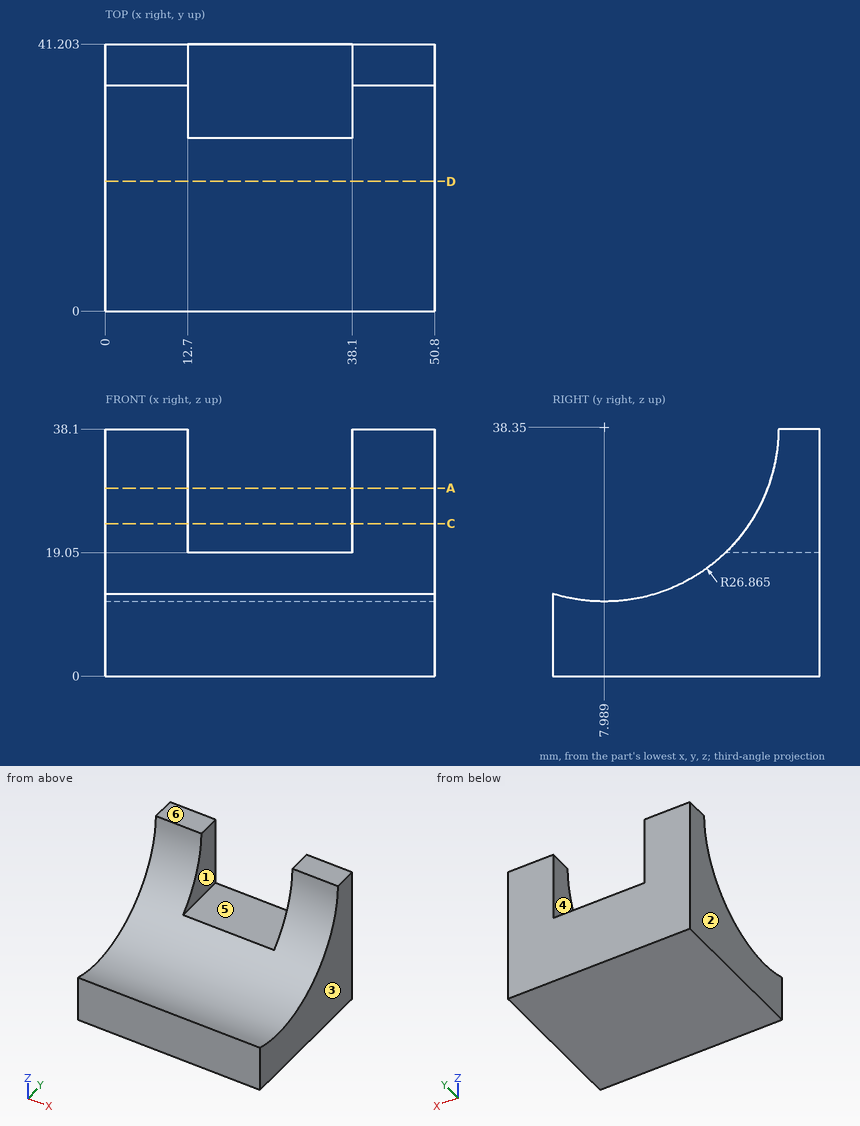
Geometry: see drawing. Coordinates: mm, zero at the bounding-box minimum. A direction names the side the tool comes from. Give positions to 0.01 mm unless a question says otherwise; leave off trailing zeros. Loops run counter-clockwise (first coordinate to the right, second up) from the corner with the lowest first, then second, coordinate; pieces in that order, holes last. Notation, with made-up numbers: M 79.5,88 L 128.5,88 A21 ccw 128.5,110 Z; hole C 67.5,24.25 d11. An arc over 180 degrees is marked long. Answer as CSV lines item,"result". Start each with the question number.
1. Pin query (flat end, axial travel): P1, Ø11.5, axis at x = 29, y = 33, coming from the +Z side. Return the tip coordinate at first contact, or that it passes through.
2. Pull-direction query (X, two-part tool) for the marked faces 3, 4, 5 and 6; classes: released by +X, released by -X, zero draft, split by the parting line, or undercut.
3. Reachability of the marked faces 1 and 2 from +Z, -Z, +X, -X, +Y, -Y: full face, straight path, thin tool, end or side. Return the list, or none.
4. Section A-A on z = 29. Return loops of the section in (x, y) (1 decimal), plus the area to 3 significant figures.
5. Line query: L1, parallel to X at y = 33, z = 26; L2, parallel to Z at x = 36, y = 33.5; L3, parallel to Z at x = 38.5, y = 7.5. Output: solid intervals per line, ascending.
6. Section C-C on z = 23.5. Return loops of the section in (x, y), plus the area to 3 significant figures.
7. Section D-D on y = 20. Return loops of the section in (x, z), plus the area to 3 significant figures.
Computed values:
1,P1,"stops at z = 19.05"
2,face 3,"released by +X"
2,face 4,"undercut"
2,face 5,"undercut"
2,face 6,"zero draft"
3,face 1,"+Z, +Y, -Y"
3,face 2,"+Z, -Z, -X, +Y, -Y"
4,outline,"M 0,33.2 L 12.7,33.2 L 12.7,41.2 L 0,41.2 Z; M 38.1,33.2 L 50.8,33.2 L 50.8,41.2 L 38.1,41.2 Z"
4,area,"204 mm²"
5,L1,"x = 0 to 12.7, 38.1 to 50.8"
5,L2,"z = 0 to 19.05"
5,L3,"z = 0 to 11.49"
6,outline,"M 0,30.38 L 12.7,30.38 L 12.7,41.2 L 0,41.2 Z; M 38.1,30.38 L 50.8,30.38 L 50.8,41.2 L 38.1,41.2 Z"
6,area,"275 mm²"
7,outline,"M 0,0 L 50.8,0 L 50.8,14.32 L 0,14.32 Z"
7,area,"727 mm²"
